Can you work these out from the model? Positions are in its coordinate system, mm. Face numbers are marked on the shaded views. A direction names the side the tool comes from. Coordinates: 2 decimals unless noted, no trailing zeros. Order: outer loops, then holes, each group sorted by start corner. A loop starts at its lowest first (then second) coordinate and runs counter-clockwise, first axis right, second up. Notation, with made-up numbers: (-5.5, 49.25) -> (2.5, 49.25) arc R17 cw to (2.5, 73.25) -> close; hole circle Ø10 at (14, 82). An arc over 180 degrees is marked (long way). Return JSON: item names as keys, results as strings. Group by question number.
1) For the marked faces 1 and 2, which set-ups out of +Z, -Z, +X, -X, +Y, -Y let a thin tool reach every point of the face, with its end or its side?
2) If we section it at B-B, the plane z = -5.75: Please give me the cut outline in (x, y).
3) If we section it at A-A, the plane z = 5: Please give me the cut outline in (x, y).
4) If we section it at C-C, the plane x = 5.5: Please give me the cut outline in (y, z).
5) If I drill on probe 1 along X at (y, z) = (-6.75, 1.5); probe 2 along Y at (x, z) = (0.5, 0.25); probe 3 along Z at (x, y) = (2, 6.5), over which ranges is the centre line in solid material (lowest first)? Write a range as from..to.
6) For pin 1 (5 mm diameter, centred on y = -5.5, z = 4, fed in from +X); pin 2 (2 mm diameter, centred on x = 6.5, z = -2, fed in from +Y); pin 3 (3 mm diameter, centred on x = 3, y = -3.5, fed in from +Z), each with a flat end and sliding along its axis, tell me the tip position at first contact or that it passes through.
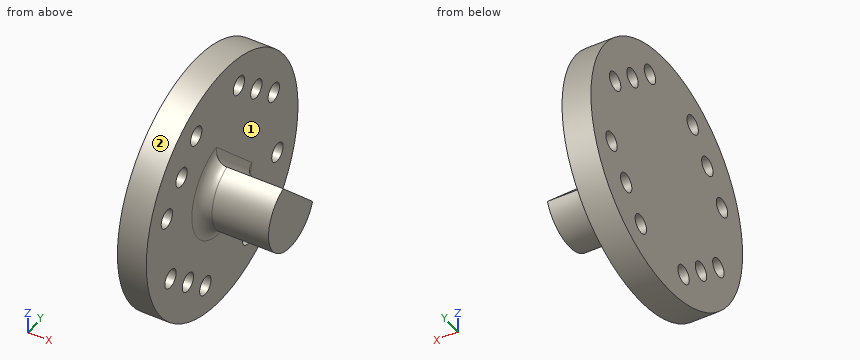
Autodesk Inventor part; units mm, degrees
ref_plane "YZ Plane" through (0, 0, 0) normal (1, 0, 0) x (0, 1, 0)
ref_plane "XZ Plane" through (0, 0, 0) normal (0, 1, 0) x (-1, 0, 0)
ref_plane "XY Plane" through (0, 0, 0) normal (0, 0, 1) x (1, 0, 0)
sketch "Sketch1" plane through (0, 0, 0) normal (1, 0, 0) x (0, 1, 0)
  circle A0 centre (0, 0) radius 10
  dimension "d0" = 20
extrude "Extrusion1" add sketch "Sketch1" along normal blind 2.3
sketch "Sketch2" plane through (2.3, 0, 0) normal (1, 0, 0) x (0, 0, -1)
  circle A0 centre (0, 0) radius 10
  circle A1 centre (-5.3514, 4.5124) radius 0.75
  circle A2 centre (-7.2853, 2.219) radius 0.75
  circle A3 centre (-4.5124, -5.3514) radius 0.75
  circle A4 centre (-2.219, -7.2853) radius 0.75
  circle A5 centre (3.4175, -6.8059) radius 0.75
  circle A6 centre (4.5124, 5.3514) radius 0.75
  circle A7 centre (2.219, 7.2853) radius 0.75
  circle A8 centre (0, 0) radius 4.4
  circle A9 centre (6.8059, 3.4175) radius 0.75
  circle A10 centre (7.2853, -2.219) radius 0.75
  circle A11 centre (5.3514, -4.5124) radius 0.75
  circle A12 centre (-6.8059, -3.4175) radius 0.75
  circle A13 centre (-3.4175, 6.8059) radius 0.75
  circle A14 centre (0, 0) radius 1.5
  point P0 (0, 0)
extrude "Extrusion2" cut sketch "Sketch2" against normal through all contours A1 | A2 | A3 | A4 | A5 | A6 | A7 | A9 | A10 | A11 | A12 | A13
sketch "Sketch3" plane through (2.3, 0, 0) normal (1, 0, 0) x (0, 0, -1)
  circle A0 centre (0, 0) radius 3
  line L0 (-4.1558, -4.1558) -> (4.1558, 4.1558) construction
  line L1 (14, 0) -> (-14, 0)
  line L2 (-2.8123, -1.0445) -> (1.0445, 2.8123)
  point P0 (-0.8839, 0.8839)
  dimension "d5" = 6
  dimension "d6" = 45
  dimension "d7" = 1.25
extrude "Extrusion3" add sketch "Sketch3" along normal blind 5.5 contours L1 L2 A0 | A0 L2 L1 picked at (1.3813, 0.2407) picked at (1.3839, -0.2301)
fillet "Fillet1" radius 1 2 edges at (2.3, 0.8839, 0.8839) (2.3, -2.1213, -2.1213)
properties part number "Printed Horn"
Result sheet:
{
 "1": {"face 1": "+X", "face 2": "+X, -X"},
 "2": {"outline": "(0, -8.18) -> (2.3, -8.18) -> (2.3, -5.15) -> (0, -5.15) -> close; (0, -3.88) -> (2.3, -3.88) -> (2.3, 8.18) -> (0, 8.18) -> close"},
 "3": {"outline": "(0, -8.66) -> (2.3, -8.66) -> (2.3, -5.92) -> (0, -5.92) -> close; (0, -4.78) -> (2.3, -4.78) -> (2.3, 3.85) -> (0, 3.85) -> close; (0, 5.17) -> (2.3, 5.17) -> (2.3, 8.66) -> (0, 8.66) -> close"},
 "4": {"outline": "(-1.04, 2.81) arc R3 ccw (long way) to (2.81, -1.04) -> close"},
 "5": {"probe 1": "x = 0..2.3", "probe 2": "y = -10..10", "probe 3": "z = -7.6..2.73, 4.1..7.6"},
 "6": {"pin 1": "stops at x = 2.3", "pin 2": "stops at y = 2.81", "pin 3": "stops at z = 9.76"}
}
